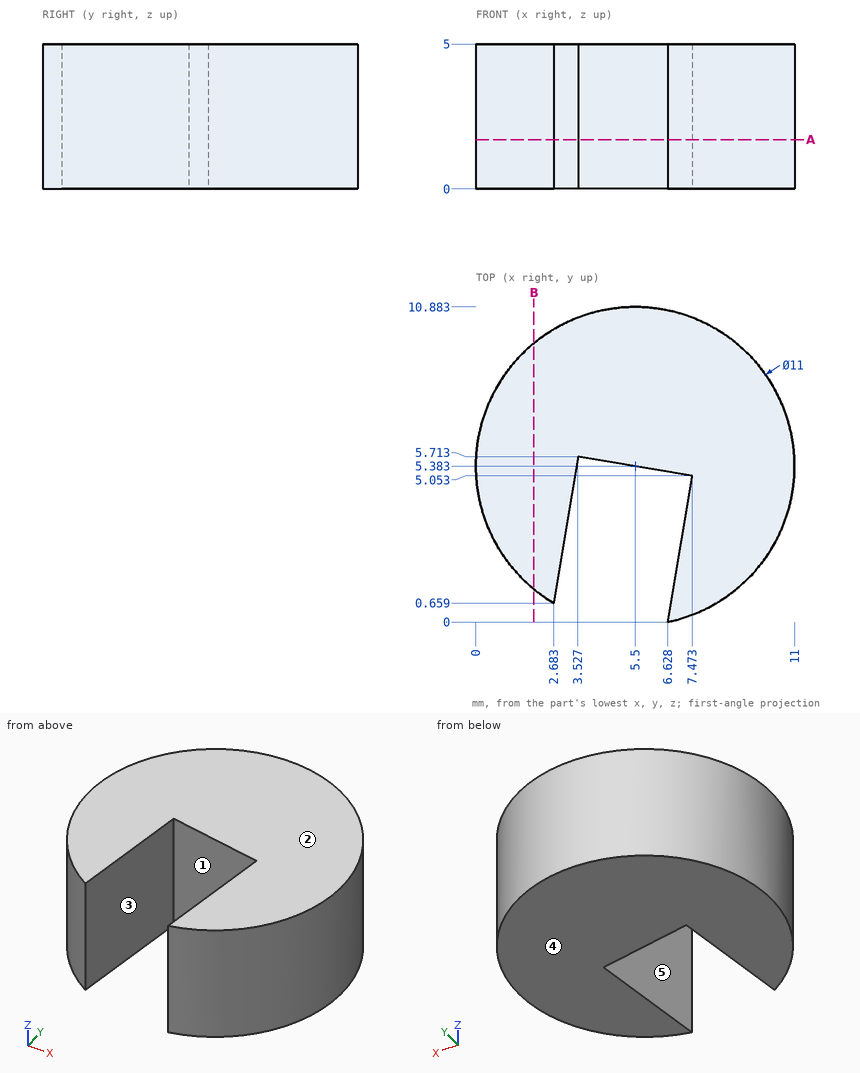
Check sheet for the drawn part. Datum: minimum x, y, z corner. Units: mm. A direction names the side the tool comes from. Round coordinates to 2 decimals unless told otherwise and drop trailing zeros. Write each loop counter-clockwise with the first axis right and the second up, starting at its lowest first coordinate (ties: lowest second). Pieces come first, ordered by that corner, then holes. Notation, with made-up numbers: (65, 25.5) - (70, 25.5) arc R19 cw to (70, 37.5) - close; hole circle Ø11 at (15, -37.5). An arc over 180 degrees is marked (long way). Write each question's results on one line, items separated by ' | '.
(1) Thickness scan on probe 1 along Y at (x, z) = (9.75, 1.65) (1 decimal); probe 2 along Y at (x, z) = (5.5, 2.15); probe 3 along X at (y, z) = (2.5, 0.5) (1 decimal). Record the ranges inside material, lowest first. Write a range as from..to.
Computed:
probe 1: y = 1.9..8.9 | probe 2: y = 5.38..10.88 | probe 3: x = 0.8..3, 7..10.2
(2) Sectioned sample at B-B, the plane x = 2. Enter the section's corners in (y, z) (1 decimal).
Computed:
outline: (1.1, 0) - (9.6, 0) - (9.6, 5) - (1.1, 5) - close
(3) Set-up check for the marked faces 4 and 5: record each of +Z, -Z, +X, -X, +Y, -Y from which the full face is reachable in a straight line by a thin tool's end or side.
Computed:
face 4: -Z, +X, -X, +Y, -Y | face 5: +Z, -Z
(4) Sectioned sample at A-A, the plane z = 1.7. Enter the section's corners in (x, y).
Computed:
outline: (2.68, 0.66) - (3.53, 5.71) - (7.47, 5.05) - (6.63, 0) arc R5.5 ccw (long way) to start
(5) Draft check along Y on the marked faces 1, 2 and 3. Enter one of: pulls with the +Y half, pulls with the -Y half, needs draft (parallel to the pull), parting line crosses it, or undercut.
Computed:
face 1: undercut | face 2: needs draft | face 3: pulls with the -Y half
